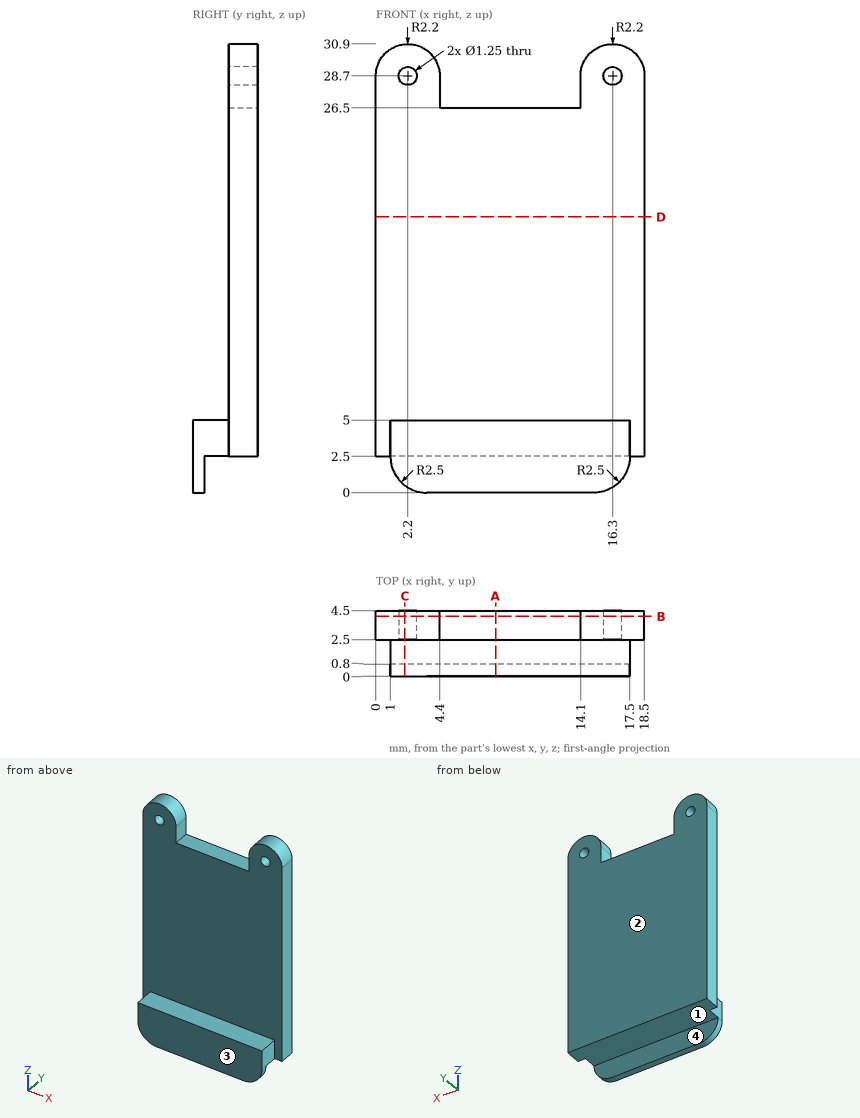
Design review of the part shown in the three views and the two pictorial views. Dimensions are in mm from the part's minimum x, y and z. A direction names the side the tool comes from. Give positions to 0.01 mm unless a question says otherwise; leave off trailing zeros. Order: outer loops, then holes, each group sorted by start corner. A loop starts at its lowest first (then second) coordinate and runs counter-clockwise, first axis right, second up. Notation, with made-up numbers: (2.25, 76) -> (61.25, 76) arc R10 cw to (61.25, 91) -> close; hole circle Ø5 at (22, 5). An arc over 180 degrees is marked (long way). Write each question's results on one line, items separated by ' | '. Start each with the question number.
Q1. For pin 1 (1.2 mm diameter, centred on y = 1.5, z = 3.5, fed in from -X); pin 2 (1.6 mm diameter, centred on x = 2.2, z = 28.7, fed in from -Y); pin 3 (0.8 mm diameter, centred on y = 0.5, z = 4, fed in from +X), all flat-tipped, find the tip position at first contact; note any pin that passes through.
Q2. Add section A-A on x = 8.25. Give the boundary of the cut face in (y, z), and give its area (4 significant figures).
Q3. Machinability: for the marked faces 3 and 4, which of the approach directions +Z, -Z, +X, -X, +Y, -Y give a long, thin tool a straight path to every point of the face, cutting with its end or side? Answer none if there is none.
Q4. Add section B-B on y = 4.1. Give the boundary of the cut face in (x, z) (3 decimals), and give its area (3 significant figures).
Q5. Add section C-C on x = 2. Give the boundary of the cut face in (y, z), and give its area (3 significant figures).
Q6. Wall thickness on L1, parallel to X at y = 3.5, z = 28.7 (3 decimals); L2, parallel to Z at x = 2.2, y = 3.3 (3 decimals); L3, parallel to Y at x = 10.25, z = 16: over which ranges is each line inside the solid? List them lowest first. Write a range as from..to.
Q7. Mouldability with a two-part tool opening along Z and no side actions: class the marked faces 1 and 2 as +Z half, -Z half, draft (parallel to the pull), parting line (faces both ways), or undercut.
Q8. Add section D-D on z = 19. Give the boundary of the cut face in (x, y).
Found:
1) pin 1: stops at x = 1 | pin 2: stops at y = 2.5 | pin 3: stops at x = 17.5
2) outline: (0, 0) -> (0.8, 0) -> (0.8, 2.5) -> (4.5, 2.5) -> (4.5, 26.5) -> (2.5, 26.5) -> (2.5, 5) -> (0, 5) -> close | area: 56.25 mm2
3) face 3: +Z, -Z, +X, -X, -Y | face 4: -Z, +X, -X, +Y
4) outline: (0, 2.5) -> (18.5, 2.5) -> (18.5, 28.7) arc R2.2 ccw to (14.1, 28.7) -> (14.1, 26.5) -> (4.4, 26.5) -> (4.4, 28.7) arc R2.2 ccw to (0, 28.7) -> close; hole circle Ø1.25 at (2.2, 28.7); hole circle Ø1.25 at (16.3, 28.7) | area: 476 mm2
5) outline: (0, 0.5) -> (0.8, 0.5) -> (0.8, 2.5) -> (4.5, 2.5) -> (4.5, 28.11) -> (2.5, 28.11) -> (2.5, 5) -> (0, 5) -> close; (2.5, 29.29) -> (4.5, 29.29) -> (4.5, 30.89) -> (2.5, 30.89) -> close | area: 62.3 mm2
6) L1: x = 0..1.575, 2.825..4.4, 14.1..15.675, 16.925..18.5 | L2: z = 2.5..28.075, 29.325..30.9 | L3: y = 2.5..4.5
7) face 1: -Z half | face 2: draft
8) outline: (0, 2.5) -> (18.5, 2.5) -> (18.5, 4.5) -> (0, 4.5) -> close
